from build123d import *

# Parameters (mm, degrees)
BOSS_EXTRUDE1_DEPTH = 40
SKETCH2_R           = 1.25
CUT_EXTRUDE1_DEPTH  = 41


with BuildPart() as part:
    # Sketch1 → Boss-Extrude1 (new body)
    with BuildSketch(Plane.XY):
        with BuildLine():
            ThreePointArc((-16.03038595, 17.148754429), (-28, 0), (-16.03038595, -17.148754429))
            ThreePointArc((-16.03038595, -17.148754429), (0, -20), (16.03038595, -17.148754429))
            ThreePointArc((16.03038595, -17.148754429), (28, 0), (16.03038595, 17.148754429))
            ThreePointArc((16.03038595, 17.148754429), (0, 20), (-16.03038595, 17.148754429))
        make_face()
    extrude(amount=BOSS_EXTRUDE1_DEPTH)

    # Sketch2 → Cut-Extrude1 (cut, through all)
    with BuildSketch(Plane.XY.offset(40)):
        with Locations((0, 10)):
            Circle(SKETCH2_R)
        with Locations((10, 0)):
            Circle(SKETCH2_R)
        with Locations((0, -10)):
            Circle(SKETCH2_R)
        with Locations((-10, 0)):
            Circle(SKETCH2_R)
        Circle(SKETCH2_R)
    extrude(amount=-CUT_EXTRUDE1_DEPTH, mode=Mode.SUBTRACT)


solid = part.part
Can you work these out from the model? Positions are in its coordinate system, mm. Give positions to 0.01 mm unless a question says otherwise; leave off trailing zeros. Order: outer loops, then holes, each group sorted by start corner. A loop starts at its lowest first (then second) coordinate and runs counter-clockwise, first axis right, second up. Notation, with made-up numbers: M 46.5,28 L 99.5,28 A14 ccw 99.5,46 Z; hole C -39,-37.5 d10. An arc over 180 degrees is marked long. Use a Markdown table: item, result. Add a question column.
Item 1: If I drill on L1, parallel to Y at x = -1, z = 13; L2, parallel to Y at x = -9, z = 33.5; L3, parallel to Y at x = -10, z = 16, over which ranges is the centre line in solid material (lowest first)? Write a range as [from, to].
Item 2: Will these pins go through, and if not, where does the flat tip stop? pin 1 (4 mm diameter, centred on x = -19.5, z = 24.5, fed in from -Y); pin 2 (10 mm diameter, centred on x = 20.5, z = 10, fed in from -Y); pin 3 (2 mm diameter, centred on x = 9, z = 27, fed in from -Y).
Item 3: We'd pull the mould along Y, two halves only. Please class faces 1 (the cylindrical face through (8.75, 0.05, 20.28)), 2 (the cylindrical face through (28, 0, 20)), 3 (the cylindrical face through (-11.25, 0.05, 20.28)), 4 (the cylindrical face through (0, 20, 20)): +Y half, -Y half, draft (parallel to the pull), parting line (faces both ways), or undercut.
Item 4: Suppose I cut it at C-C (y = -10). List the corners of the cut face in (x, z) for me, then the cut area to 3 significant figures.
Item 5: Suppose I cut it at B-B (z = 15). List the corners of the cut face in (x, y) for me, then the cut area to 3 significant figures.
Item 6: Suppose I cut it at A-A (x = 0). List the corners of the cut face in (y, z) for me.
Item 7: Suppose I cut it at D-D (x = 10). List the corners of the cut face in (y, z) for me.
Answer sheet:
| question | item | result |
|---|---|---|
| 1 | L1 | y = [-19.99, -10.75], [-9.25, -0.75], [0.75, 9.25], [10.75, 19.99] |
| 1 | L2 | y = [-19.12, -0.75], [0.75, 19.12] |
| 1 | L3 | y = [-18.91, -1.25], [1.25, 18.91] |
| 2 | pin 1 | stops at y = -16.53 |
| 2 | pin 2 | stops at y = -17.34 |
| 2 | pin 3 | stops at y = -19.31 |
| 3 | face 1 | undercut |
| 3 | face 2 | parting line |
| 3 | face 3 | undercut |
| 3 | face 4 | +Y half |
| 4 | outline | M -25.02,0 L -1.25,0 L -1.25,40 L -25.02,40 Z; M 1.25,0 L 25.02,0 L 25.02,40 L 1.25,40 Z |
| 4 | area | 1,900 mm² |
| 5 | outline | M -16.03,-17.15 A46.49 ccw 16.03,-17.15 A18.27 ccw 16.03,17.15 A46.49 ccw -16.03,17.15 A18.27 ccw Z; hole C -10,0 d2.5; hole C 0,-10 d2.5; hole C 0,0 d2.5; hole C 0,10 d2.5; hole C 10,0 d2.5 |
| 5 | area | 1,800 mm² |
| 6 | outline | M -20,0 L -11.25,0 L -11.25,40 L -20,40 Z; M -8.75,0 L -1.25,0 L -1.25,40 L -8.75,40 Z; M 1.25,0 L 8.75,0 L 8.75,40 L 1.25,40 Z; M 11.25,0 L 20,0 L 20,40 L 11.25,40 Z |
| 7 | outline | M -18.91,0 L -1.25,0 L -1.25,40 L -18.91,40 Z; M 1.25,0 L 18.91,0 L 18.91,40 L 1.25,40 Z |
